Geometry check sheet. Reference: the model listing, model coordinates, mm. A direction names the side the tool comes from. Give positions to 0.01 mm unless a question says otherwise; leave off trailing zeros. Order: outer loops, then holes, each group sorted by start corner. A loop starts at its lowest first (then second) coordinate and runs counter-clockwise, first axis right, second up. Notation, with made-up numbers: (35, 42) - (49, 42) arc R35 cw to (49, 79) - close; hole circle Ø7 at (49, -21.75). An arc over 180 degrees is marked (long way). Put each result on its own line as item: value. Start each with the question number.
```python
from build123d import *

# Parameters (mm, degrees)
ESQUISSE1_W                                        = 90
ESQUISSE1_H                                        = 90
BOSS_EXTRU_1_DEPTH                                 = 15
ESQUISSE2_R                                        = 41
BOSS_EXTRU_2_DEPTH                                 = 52
CHANFREIN1_SIZE                                    = 3
CONG_1_R                                           = 2
CHANFREIN2_SIZE                                    = 2
CHAMBRAGE_POUR_VIS_T_TE_HEXAGONALE_M41_D           = 4.5
CHAMBRAGE_POUR_VIS_T_TE_HEXAGONALE_M41_CBORE_D     = 8
CHAMBRAGE_POUR_VIS_T_TE_HEXAGONALE_M41_CBORE_DEPTH = 4.4
ESQUISSE6_R                                        = 32.5
ENL_V_MAT_EXTRU_1_DEPTH                            = 93.406709713


with BuildPart() as part:
    # Esquisse1 → Boss.-Extru.1 (new body)
    with BuildSketch(Plane(origin=(0, 0, 0), x_dir=(1, 0, 0), z_dir=(0, 1, 0))):
        Rectangle(ESQUISSE1_W, ESQUISSE1_H)
    extrude(amount=BOSS_EXTRU_1_DEPTH)

    # Esquisse2 → Boss.-Extru.2 (add)
    with BuildSketch(Plane(origin=(0, 15, 0), x_dir=(1, 0, 0), z_dir=(0, 1, 0))):
        with Locations(Location((0, 0, 0), (0, 0, 90))):
            Circle(ESQUISSE2_R)
    extrude(amount=BOSS_EXTRU_2_DEPTH)

    # Chanfrein1
    chanfrein1_edges = [part.edges().sort_by_distance(p)[0] for p in [
        (0, 15, -45),
        (0, 15, 45),
    ]]
    chamfer(chanfrein1_edges, length=CHANFREIN1_SIZE)

    # Congé1
    cong_1_edges = [part.edges().sort_by_distance(p)[0] for p in [
        (-45, 6, 45),
        (-45, 6, -45),
        (45, 6, -45),
        (45, 6, 45),
    ]]
    fillet(cong_1_edges, radius=CONG_1_R)

    # Chanfrein2
    chanfrein2_edges = [part.edges().sort_by_distance(p)[0] for p in [
        (0, 67, 41),
    ]]
    chamfer(chanfrein2_edges, length=CHANFREIN2_SIZE)

    # Chambrage pour vis à tête hexagonale M41 (through all)
    with Locations(Plane(origin=(0, 15, 0), x_dir=(1, 0, 0), z_dir=(0, 1, 0))):
        with Locations((-35, 36.5), (35, 36.5), (-35, -36.5), (35, -36.5)):
            CounterBoreHole(CHAMBRAGE_POUR_VIS_T_TE_HEXAGONALE_M41_D / 2, CHAMBRAGE_POUR_VIS_T_TE_HEXAGONALE_M41_CBORE_D / 2, CHAMBRAGE_POUR_VIS_T_TE_HEXAGONALE_M41_CBORE_DEPTH)

    # Esquisse6 → Enlèv. mat.-Extru.1 (cut, through all)
    with BuildSketch(Plane(origin=(0, 67, 0), x_dir=(1, 0, 0), z_dir=(0, 1, 0))):
        with Locations(Location((0, 0, 0), (0, 0, 270))):
            Circle(ESQUISSE6_R)
    extrude(amount=-ENL_V_MAT_EXTRU_1_DEPTH, mode=Mode.SUBTRACT)


solid = part.part
```
Item 1: Cross-section at A-A (y = 5). Enter the section's corners in (x, z).
Item 2: Cross-section at B-B (x = 0). Enter the section's corners in (y, z), and give its area (3 significant figures).
Item 3: Set-up check for faces 4 (the face through (-36.21, 5.226, 34.603)), 5 (the face through (-33, 10.6, -35)): record each of +Z, -Z, +X, -X, +Y, -Y from which the full face is reachable in a straight line by a thin tool's end or side.
Item 4: Cross-section at C-C (z = -36.5). Count the separate pieces of the cut face and the enclosed holes in it, and give its area (3 significant figures).
Item 5: Release check for a two-part mould opening along X. For faces 1 (the face through (37, 10.6, 38)), 2 (the face through (40, 40, 9)), 3 (the face through (-32, 67, 9)) record: +X half, -X half, draft (parallel to the pull), parting line (faces both ways), or undercut.
Item 6: Gauge pin test, flat ends, axial feed: pin 1 Ø5 at (x, y) = (-1, 32.5) entering from -Z; pin 2 Ø1 at (y, z) = (48.5, 33.5) entering from +X; pin 3 Ø4 at (y, z) = (31, 21.5) entering from -X. Record the tip position at first contact, or that the pin passes through.
Item 7: Thickness scan on line 1 along Z through (x, y) = (-35, 5.5); line 2 along X through (y, z) = (13, -36.5); line 3 along Z through (x, y) = (-35, 13.85). Record the ranges inside material, lowest first.
Item 8: Cross-section at D-D (y = 26). Enter the section's corners in (x, z).
Recorded:
1. outline: (-45, -43) arc R2 ccw to (-43, -45) - (43, -45) arc R2 ccw to (45, -43) - (45, 43) arc R2 ccw to (43, 45) - (-43, 45) arc R2 ccw to (-45, 43) - close; hole circle Ø4.5 at (-35, -36.5); hole circle Ø4.5 at (-35, 36.5); hole circle Ø65 at (0, 0); hole circle Ø4.5 at (35, -36.5); hole circle Ø4.5 at (35, 36.5)
2. outline: (0, -45) - (12, -45) - (15, -42) - (15, -41) - (65, -41) - (67, -39) - (67, -32.5) - (0, -32.5) - close; (0, 32.5) - (67, 32.5) - (67, 39) - (65, 41) - (15, 41) - (15, 42) - (12, 45) - (0, 45) - close
2. area: 1,250 mm^2
3. face 4: +Y, -Y
3. face 5: +Y
4. separate pieces: 3
4. enclosed holes: 0
4. area: 3,120 mm^2
5. face 1: undercut
5. face 2: parting line
5. face 3: draft
6. pin 1: stops at z = -41
6. pin 2: stops at x = 24.33
6. pin 3: stops at x = -36.07
7. line 1: z = -45 to -38.75, -34.25 to 34.25, 38.75 to 45
7. line 2: x = -45 to -39, -31 to 31, 39 to 45
7. line 3: z = -43.15 to -40.5, -32.5 to 32.5, 40.5 to 43.15
8. outline: circle Ø82 at (0, 0); hole circle Ø65 at (0, 0)
